from build123d import *

# Parameters (mm, degrees)
F0_W     = 824
F0_H     = 2000
F1_DEPTH = 50
F2_W     = 650
F2_H     = 210
F2_W_2   = 230
F2_H_2   = 1166
F3_DEPTH = 20
F4_SIZE  = 19.99999


# Not quite as in the source:
# - a fillet or chamfer is up to 0.001 mm smaller than in the source, because OpenCascade refuses the exact size


with BuildPart() as f1:
    # F0 (on Front) → F1 (new body)
    with BuildSketch(Plane.XZ):
        Rectangle(F0_W, F0_H)
    extrude(amount=F1_DEPTH)

    # F2 (on face) → F3 (cut)
    with BuildSketch(Plane.XZ.offset(50)):
        with Locations((0, 775)):
            Rectangle(F2_W, F2_H)
        with Locations((-210, 0)):
            Rectangle(F2_W_2, F2_H_2)
        with Locations((210, 0)):
            Rectangle(F2_W_2, F2_H_2)
        with Locations((0, -775)):
            Rectangle(F2_W, F2_H)
    extrude(amount=-F3_DEPTH, mode=Mode.SUBTRACT)

    # F4 (size 20 in the source; OpenCascade refuses exactly that, so slightly less here)
    f4_edges = [f1.edges().sort_by_distance(p)[0] for p in [
        (-95, -30, 0),
        (-210, -30, 583),
        (-325, -30, 0),
        (-210, -30, -583),
        (210, -30, -583),
        (95, -30, 0),
        (325, -30, 0),
        (210, -30, 583),
        (0, -30, 880),
        (-325, -30, 775),
        (325, -30, 775),
        (0, -30, 670),
        (-325, -30, -775),
        (0, -30, -880),
        (325, -30, -775),
        (0, -30, -670),
    ]]
    chamfer(f4_edges, length=F4_SIZE)


solid = f1.part
Part model, mm, in its own coordinate system. A direction names the side the tool comes from. Coordinates: 2 decimals unless noted, no trailing zeros. Use a Markdown table: item, result. Add a question column.
Q1. Which spindle directions (+Z, -Z, +X, -X, +Y, -Y) get a long thin tool onto all of the face, cutting with end or side? Do faces 1 (the flat face through (-4, -30, -774)), 2 (the flat face through (-6, 0, 14)). Say none if no direction does.
Q2. Probe L1, parallel to X at y = -33.5, z = -172.5; L2, parallel to Z at x = -202, y = -43; L3, parallel to Z at x = 27, y = -34.5. List the from-to ranges inside material, lowest first.
Q3. Mould opens along X. For faces 3 (the flat face through (412, -25, -14)), 4 (the flat face through (-412, -25, -14)), 5 (the flat face through (-4, -30, 776)) say: +X half, -X half, draft (parallel to the pull), parting line (faces both ways), or undercut.
Q4. Pin check, flat tip, straight feed: P1, Ø5, axis at x = 80.5, z = -774.5, coming from the -Y side. Stop position of the tip, or through.
Worked out:
| question | item | result |
|---|---|---|
| 1 | face 1 | -Y |
| 1 | face 2 | +Z, -Z, +X, -X, +Y |
| 2 | L1 | x = -412 to -308.5, -111.5 to 111.5, 308.5 to 412 |
| 2 | L2 | z = -1000 to -873, -677 to -576, 576 to 677, 873 to 1000 |
| 2 | L3 | z = -1000 to -864.5, -685.5 to 685.5, 864.5 to 1000 |
| 3 | face 3 | +X half |
| 3 | face 4 | -X half |
| 3 | face 5 | undercut |
| 4 | P1 | stops at y = -30 |
